```python
from build123d import *

# Parameters (mm, degrees)
CUT_EXTRUDE_1_DEPTH = 1.3
FILLET_1_R          = 0.2


with BuildPart() as part:
    # 草图1 → 旋转1 (revolve)
    with BuildSketch(Plane.XY):
        Polygon((0, 0), (0, 2.84), (3, 2.84), (3, 1.49), (31, 1.49), (31, 0), align=None)
    revolve(axis=Axis((0, 0, 0), (1, 0, 0)))

    # 草图2 → 切除-拉伸1 (cut)
    with BuildSketch(Plane.ZY):
        Polygon((-1.443375673, 0), (-0.721687836, -1.25), (0.721687836, -1.25), (1.443375673, 0), (0.721687836, 1.25), (-0.721687836, 1.25), align=None)
    extrude(amount=-CUT_EXTRUDE_1_DEPTH, mode=Mode.SUBTRACT)

    # 圆角1
    fillet_1_edges = [part.edges().sort_by_distance(p)[0] for p in [
        (0, -2.84, 0),
    ]]
    fillet(fillet_1_edges, radius=FILLET_1_R)


solid = part.part
```
Source: CAD feature listing. Evaluate the final solid. Frame: model axes, mm. A direction names the side the tool comes from. Coordinates: 2 decimals unless noted, no trailing zeros. Loops run counter-clockwise (first coordinate to the right, second up) from the corner with the lowest first, then second, coordinate; pieces in that order, holes last. Notation, with made-up numbers: M 49.25,1.5 L 85.25,1.5 A20 cw 85.25,28.5 Z; hole C 72,34 d7. An arc over 180 degrees is marked long. Use a Markdown table: item, result. Add a question column.
Q1. Draft query along Z for faces 4 (the flat face through (0.641, -0.616, -1.088)), 5 (the flat face through (31, 0, 0)), 6 (the cylindrical face through (17.196, -0.194, 1.477)). Return one class per face: pulls with the +Z half, pulls with the -Z half, needs draft (parallel to the pull), parting line crosses it, or undercut.
Q2. Section query B-B, the plane x = 21. Return loops of the section in (y, z).
Q3. Access query for faces 1 (the flat face through (0, -1.1, -1.1)), 2 (the flat face through (3, 1.2, -1.2)), 3 (the flat face through (0.641, 0.616, 1.088)). Directions: +Z, -Z, +X, -X, +Y, -Y. A direction counts if a zero-diameter tool reaches every point of the face in a straight line with its end or side. Return the directions, or none.
Q4. Section query A-A, the plane z = 0. Return loops of the section in (x, y), and give its area (3 significant figures).
Q5. First-contact query: pin 1 (1 mm diameter, centred on x = 26.5, z = -1.5, fed in from -Y); pin 2 (1.5 mm diameter, centred on x = 9, z = 1, fed in from -Y). Flat tips, straight axial feed; report the tip coordinate or a pass-through.
Q6. Material intervals for L1, parallel to X at y = 0.55, z = -2; L2, parallel to X at y = 1.2, z = 0.5; L3, parallel to Z at x = 11.5, y = 0.05, sorted ascending.
Result:
| question | item | result |
|---|---|---|
| 1 | face 4 | undercut |
| 1 | face 5 | needs draft |
| 1 | face 6 | parting line crosses it |
| 2 | outline | C 0,0 d2.98 |
| 3 | face 1 | +Z, -Z, -X, +Y, -Y |
| 3 | face 2 | +X |
| 3 | face 3 | -X |
| 4 | outline | M 0,-2.64 A0.2 ccw 0.2,-2.84 L 3,-2.84 L 3,-1.49 L 31,-1.49 L 31,1.49 L 3,1.49 L 3,2.84 L 0.2,2.84 A0.2 ccw 0,2.64 L 0,1.25 L 1.3,1.25 L 1.3,-1.25 L 0,-1.25 Z |
| 4 | area | 97.2 mm2 |
| 5 | pin 1 | stops at y = -1.1 |
| 5 | pin 2 | stops at y = -1.47 |
| 6 | L1 | x = 0 to 3 |
| 6 | L2 | x = 1.3 to 31 |
| 6 | L3 | z = -1.49 to 1.49 |
